Could you check a few things on this model? Use its own coordinates, in mm. Round coordinates to 2 decimals unless told otherwise and drop trailing zeros. Loops run counter-clockwise (first coordinate to the right, second up) from the corner with the lowest first, then second, coordinate; pieces in that order, holes last.
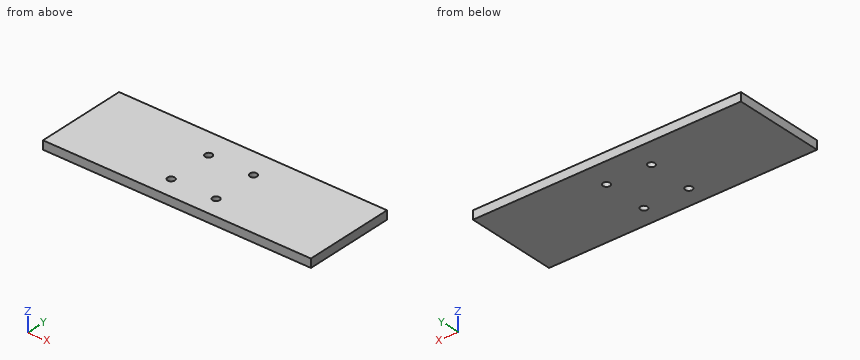
from build123d import *

# Parameters (mm, degrees)
SKETCH1_W           = 596.9
SKETCH1_H           = 203.2
BOSS_EXTRUDE1_DEPTH = 9.525
SKETCH2_R           = 7.9375
CUT_EXTRUDE1_DEPTH  = 20.05


with BuildPart() as part:
    # Sketch1 → Boss-Extrude1 (new body, symmetric)
    with BuildSketch(Plane.XY):
        Rectangle(SKETCH1_W, SKETCH1_H)
    extrude(amount=BOSS_EXTRUDE1_DEPTH, both=True)

    # Sketch2 → Cut-Extrude1 (cut, through all)
    with BuildSketch(Plane.XY.offset(9.525)):
        with Locations((-50, 42.85)):
            Circle(SKETCH2_R)
        with Locations((-50, -57.15)):
            Circle(SKETCH2_R)
        with Locations((50, 42.85)):
            Circle(SKETCH2_R)
        with Locations((50, -57.15)):
            Circle(SKETCH2_R)
    extrude(amount=-CUT_EXTRUDE1_DEPTH, mode=Mode.SUBTRACT)


solid = part.part
Item 1: If I drill on line 1 along Y through (x, z) = (-50, 3.25); line 2 along X through (y, z) = (-59.5, 5.75); line 3 along X through (y, z) = (36, 8.5), over which ranges is the centre line in solid material (lowest first)?
Results list:
line 1: y = -101.6 to -65.09, -49.21 to 34.91, 50.79 to 101.6
line 2: x = -298.45 to -57.58, -42.42 to 42.42, 57.58 to 298.45
line 3: x = -298.45 to -54.01, -45.99 to 45.99, 54.01 to 298.45
Item 2: If we section it at B-B, the plane y = 42.85: Count the separate pieces of the cut face and the enclosed holes in it, then the cut area to 3 significant figures.
Results list:
separate pieces: 3
enclosed holes: 0
area: 10,800 mm2
Item 3: If we section it at A-A, the plane x = 50: Please give me the cut outline in (y, z) (1 decimal), then the cut area to 3 significant figures.
Results list:
outline: (-101.6, -9.5) - (-65.1, -9.5) - (-65.1, 9.5) - (-101.6, 9.5) - close; (-49.2, -9.5) - (34.9, -9.5) - (34.9, 9.5) - (-49.2, 9.5) - close; (50.8, -9.5) - (101.6, -9.5) - (101.6, 9.5) - (50.8, 9.5) - close
area: 3,270 mm2
